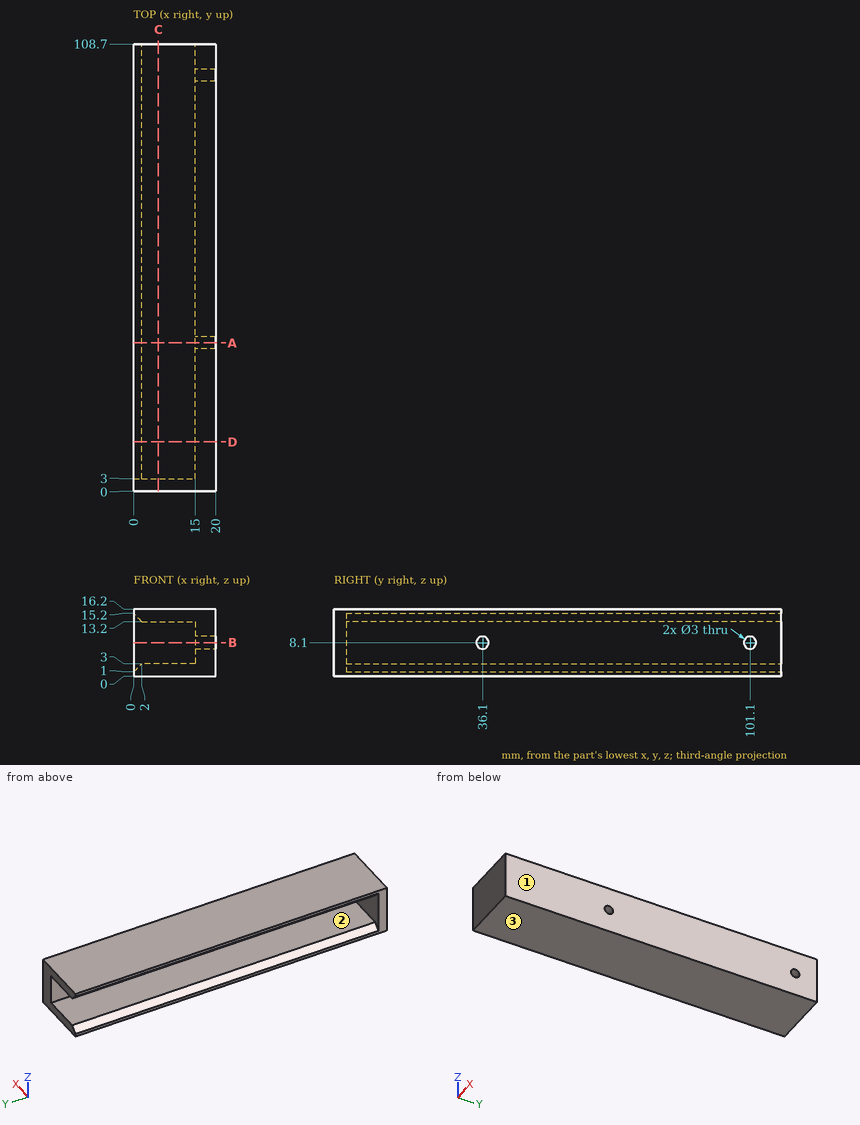
Job drawing, mm, ordinate dimensions from the low corner. One solid piece. Give positions to 0.01 mm unless a question says otherwise; leave off trailing zeros. Loops run counter-clockwise (first coordinate to the right, second up) from the corner with the lowest first, then second, coordinate; pieces in that order, holes last. Notation, with made-up numbers: M -20.5,36 L 32.5,36 A28 ccw 32.5,70 Z; hole C 73,52 d2. An arc over 180 degrees is marked long. Return JSON: item names as keys, results as strings.
1) Saw through at A-A, the plane y = 36.1. List the corners of the cut face in (x, z).
Calculated:
{"outline": "M 0,0 L 20,0 L 20,6.6 L 15,6.6 L 15,3 L 2,3 L 0,1 Z; M 0,15.2 L 2,13.2 L 15,13.2 L 15,9.6 L 20,9.6 L 20,16.2 L 0,16.2 Z"}
2) Pull direction Z, two halves, no side cores. Call the marked faces 1, 2 and 3: released by +Z, released by -Z, zero draft, split by the parting line, or undercut.
Calculated:
{"face 1": "zero draft", "face 2": "undercut", "face 3": "released by -Z"}
3) Flat gauge pins, fed straight in: pin 1 Ø3 at (x, y) = (17.5, 93) entering from -Z; pin 2 Ø8 at (y, z) = (77, 8) entering from -X; pin 3 Ø2 at (y, z) = (66.5, 13) entering from -X; pin 4 Ø3 at (x, z) = (3, 10.5) entering from +Y. Where does each tip first touch, or does it go through?
Calculated:
{"pin 1": "stops at z = 0", "pin 2": "stops at x = 15", "pin 3": "stops at x = 1.2", "pin 4": "stops at y = 3"}
4) Saw through at B-B, the plane z = 8.1. List the corners of the cut face in (x, y), then the cut area to 4 significant figures.
Calculated:
{"outline": "M 0,0 L 20,0 L 20,34.6 L 15,34.6 L 15,3 L 0,3 Z; M 15,37.6 L 20,37.6 L 20,99.6 L 15,99.6 Z; M 15,102.6 L 20,102.6 L 20,108.7 L 15,108.7 Z", "area": "558.5 mm2"}
5) Saw through at C-C, the plane x = 6. List the corners of the cut face in (y, z), then the cut area to 3 significant figures.
Calculated:
{"outline": "M 0,0 L 108.7,0 L 108.7,3 L 3,3 L 3,13.2 L 108.7,13.2 L 108.7,16.2 L 0,16.2 Z", "area": "683 mm2"}
6) Saw through at D-D, the plane y = 12. List the corners of the cut face in (x, z), then the cut area to 3 significant figures.
Calculated:
{"outline": "M 0,0 L 20,0 L 20,16.2 L 0,16.2 L 0,15.2 L 2,13.2 L 15,13.2 L 15,3 L 2,3 L 0,1 Z", "area": "167 mm2"}
7) Drill centre lines: line 1 (Y direction, x = 18, z = 8.1); line 2 (Z direction, x = 17.3, y = 101.1); line 3 (Z direction, x = 6, y = 15.5). Where is each one in solid material? Low to high.
Calculated:
{"line 1": "y = 0 to 34.6, 37.6 to 99.6, 102.6 to 108.7", "line 2": "z = 0 to 6.6, 9.6 to 16.2", "line 3": "z = 0 to 3, 13.2 to 16.2"}
